Check sheet for the modelled part. Datum: model origin and axes. Units: mm. Face numbers are marked on the shaded views. A direction names the side the tool comes from. Round coordinates to 2 decimals unless told otherwise and drop trailing zeros. Order: outer loops, then holes, each group sorted by start corner. A loop starts at its lowest first (then second) coordinate and runs counter-clockwise, first axis right, second up.
```python
from build123d import *

# Parameters (mm, degrees)
F0_W     = 70
F0_H     = 77
F1_DEPTH = 29.4
F2_W     = 25.4
F2_H     = 66
F3_DEPTH = 75
F5_DEPTH = 70
F6_R     = 0.9
F7_DEPTH = 70
F8_DEPTH = 70


with BuildPart() as f1:
    # F0 (on Right) → F1 (new body)
    with BuildSketch(Plane.YZ):
        with Locations((35, 38.5)):
            Rectangle(F0_W, F0_H)
    extrude(amount=F1_DEPTH)

    # F2 (on Top) → F3 (cut)
    with BuildSketch(Plane.XY):
        with Locations((14.7, 35)):
            Rectangle(F2_W, F2_H)
    extrude(amount=F3_DEPTH, mode=Mode.SUBTRACT)

    # F4 (on face) → F5 (cut, through all)
    with BuildSketch(Plane(origin=(0, 70, 0), x_dir=(-1, 0, 0), z_dir=(0, 1, 0))):
        Polygon((0, 0), (0, 12), (-29.4, 0), align=None)
    extrude(amount=-F5_DEPTH, mode=Mode.SUBTRACT)

    # F6 (on face) → F7 (join)
    with BuildSketch(Plane(origin=(0, 70, 0), x_dir=(-1, 0, 0), z_dir=(0, 1, 0))):
        with BuildLine():
            ThreePointArc((-33.1859084974, 0.2855383414), (-31.8851667844, 2.4284246469), (-29.4, 2.7568097504))
            Line((-29.4, 2.7568097504), (-29.4, 77))
            Line((-29.4, 77), (-33.1859084974, 0.2855383414))
        make_face()
        with BuildLine():
            Line((-27.5050449892, 0.7734510248), (-29.4, 0))
            Line((-29.4, 0), (-29.4, 2.7568097504))
            ThreePointArc((-29.4, 2.7568097504), (-31.8851667844, 2.4284246469), (-33.1859084974, 0.2855383414))
            Line((-33.1859084974, 0.2855383414), (-33.2, 0))
            ThreePointArc((-33.2, 0), (-30.3, -2.9), (-27.4, 0))
            ThreePointArc((-27.4, 0), (-27.4263812421, 0.390275844), (-27.5050449892, 0.7734510248))
        make_face()
        with Locations((-30.3, 0)):
            Circle(F6_R, mode=Mode.SUBTRACT)
        with Locations((-30.3, 0)):
            Circle(F6_R)
    extrude(amount=-F7_DEPTH)

    # F6 (on face) → F8 (cut, through all)
    with BuildSketch(Plane(origin=(0, 70, 0), x_dir=(-1, 0, 0), z_dir=(0, 1, 0))):
        with Locations((-30.3, 0)):
            Circle(F6_R)
    extrude(amount=-F8_DEPTH, mode=Mode.SUBTRACT)


solid = f1.part
```
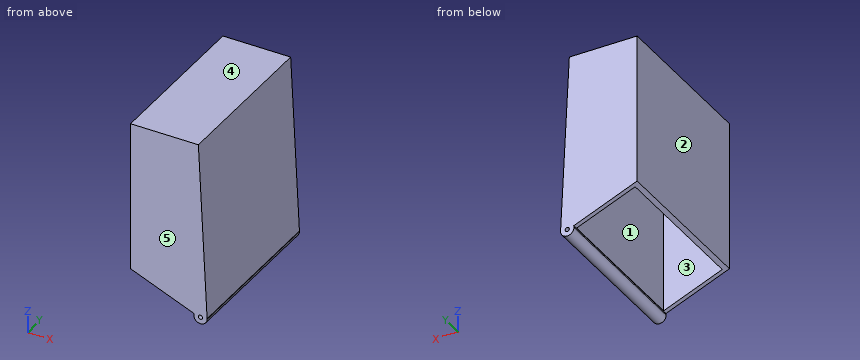
Item 1: Go/stop test with flat-tipped pins: P1, Ø4, axis at x = 15, y = 38, coming from the -Z side; P2, Ø4, axis at y = 49, z = 10.5, coming from the +X side; P3, Ø8, axis at y = 23.5, z = 31.5, coming from the +X side. Record where each tip stops, or that it passes through.
Answer:
P1: stops at z = 75
P2: stops at x = 32.78
P3: stops at x = 31.84
Item 2: Access from +Z, -Z, +X, -X, +Y, -Y to the whole of each face (thin tool, end or side, straight path). Record for the marked faces 1 and 2.
Answer:
face 1: -Z
face 2: +Z, -Z, -X, +Y, -Y
Item 3: Sectioned sample at B-B (x = 30.3). Record the cut outline in (y, z), and give its area (3 significant figures).
Answer:
outline: (0, -2.9) - (70, -2.9) - (70, -0.9) - (0, -0.9) - close; (0, 0.9) - (70, 0.9) - (70, 58.76) - (0, 58.76) - close
area: 4,190 mm2
Item 4: Sectioned sample at D-D (x = 7.5). Record the cut outline in (y, z).
Answer:
outline: (0, 8.94) - (2, 8.94) - (2, 75) - (68, 75) - (68, 8.94) - (70, 8.94) - (70, 77) - (0, 77) - close
Item 5: Sectioned sample at C-C (z = 21). Record the cut outline in (x, y), and give its area (3 significant figures).
Answer:
outline: (0, 0) - (32.16, 0) - (32.16, 70) - (0, 70) - close; hole (2, 2) - (27.4, 2) - (27.4, 68) - (2, 68) - close
area: 575 mm2
Item 6: Scan lines: line 1 along Y through (x, z) = (16, 63); line 2 along Z through (x, y) = (10.5, 19); line 3 along X through (y, z) = (43, 47). Record each from-to range of solid material in increasing order.
Answer:
line 1: y = 0 to 2, 68 to 70
line 2: z = 75 to 77
line 3: x = 0 to 2, 27.4 to 30.88
Item 7: Release check for a two-part mould opening along Y. For the marked faces 3, 4 and 5 record: released by +Y, released by -Y, zero draft, split by the parting line, or undercut.
Answer:
face 3: undercut
face 4: zero draft
face 5: released by -Y
Item 8: Sectioned sample at A-A (y = 19.5). Record the cut outline in (x, z).
Answer:
outline: (0, 12) - (2, 11.18) - (2, 75) - (27.4, 75) - (27.4, 0.82) - (27.51, 0.77) arc R2.9 ccw (long way) to (33.2, 0) - (29.4, 77) - (0, 77) - close; hole circle Ø1.8 at (30.3, 0)
